Input: part model. Units: mm. Frame: model coordinates. A direction names the side the tool comes from. Give positions to 0.01 mm unless a question says otherwise; leave off trailing zeros. Write each loop counter-clockwise with the first axis right and the second up, starting at its lowest first coordinate (ties: lowest second). Pieces come first, ordered by that corner, then holes. Notation, with made-up numbers: (62.5, -22.75) -> (94.5, -22.75) arc R29 ccw to (94.5, 13.25) -> close; hole circle Ø1 at (72.25, 51.25). An arc over 180 degrees is marked (long way). Return JSON: item names as keys, results as strings. Group by question number.
Item 1: Line query: line 1 (X direction, y = 0, z = 25); line 2 (X direction, y = 29.5, z = 1); line 3 (X direction, y = 0, z = 15). Output: solid intervals per line, ascending. Write a range as [from, to].
Item 2: Set-up query: faces 4 (the face through (33.79, 0.41, -3.15)), 5 (the face through (39.962, -17, -17)), 6 (the face through (31.618, -17, 17)). Return all of +Z, -Z, +X, -X, +Y, -Y with unobstructed straight access to the full face (end or side cutting, diameter ignored); none if empty.
Item 3: Section C-C, the plane x = 47. Return loops of the section in (y, z) (3 decimals).
Item 4: Section B-B, the plane x = 28.5. Return loops of the section in (y, z) (3 decimals).
Item 5: Mould query, pull axis X, two halves, no side actions, for faces 1 (the face through (26.68, 13.65, -14.89)), 2 (the face through (38.82, -0.95, 19.44)), 3 (the face through (11.521, -10.465, -2.324)). Classes: released by +X, released by -X, zero draft, split by the parting line, or undercut.
Item 6: Section D-D, the plane y = -26. Return loops of the section in (x, z), then the cut area to 3 significant figures.
Item 7: Section A-A, the plane y = 0. Return loops of the section in (x, z) (1 decimal).
Item 8: Pin query (flat end, axial travel): P1, Ø8, axis at x = 30, z = -4, coming from the +Y side; P2, Ø1, axis at x = 38.5, y = -30.5, coming from the -Z side; P3, Ø2, axis at x = 51, z = -2, coming from the +Y side. Return the tip coordinate at first contact, or that it passes through.
from build123d import *

# Parameters (mm, degrees)
F4_D     = 6.35
F4_DEPTH = 39.4386441836
F5_D     = 6.35


with BuildPart() as f1:
    # F0 (on Front) → F1 (revolve)
    with BuildSketch(Plane.XZ):
        Polygon((10.9917372465, 10.2357640862), (10.9917372465, 0), (55.9533685446, 0), (55.9533685446, 10.2357640862), (39.9618595839, 21.1285278201), (39.9618595839, 39.4376441836), (31.6184610128, 39.4376441836), (31.6184610128, 20.2014818788), (21.8845009804, 20.2014818788), align=None)
    revolve(axis=Axis((33.4725528955, 0, 0), (-1, 0, 0)))

    # F4 (through all, one way)
    with BuildSketch(Plane(origin=(0, 0, 0), x_dir=(1, 0, 0), z_dir=(0, 0, -1))):
        with Locations((35.7924923301, 0)):
            Circle(F4_D / 2)
    extrude(amount=-F4_DEPTH, mode=Mode.SUBTRACT)

    # F5 (through all)
    with Locations(Plane(origin=(0, 0, 0), x_dir=(0, 1, 0), z_dir=(-1, 0, 0))):
        with Locations((0, 0)):
            Hole(F5_D / 2)


solid = f1.part
Answer below:
{
 "1": {"line 1": "x = [31.62, 32.62], [38.97, 39.96]", "line 2": "x = [31.62, 39.96]", "line 3": "x = [16.2, 32.62], [38.97, 48.96]"},
 "2": {"face 4": "+X, -X", "face 5": "+X", "face 6": "-X"},
 "3": {"outline": "circle Ø32.669 at (0, 0); hole circle Ø6.35 at (0, 0)"},
 "4": {"outline": "circle Ø40.403 at (0, 0); hole circle Ø6.35 at (0, 0)"},
 "5": {"face 1": "zero draft", "face 2": "undercut", "face 3": "released by -X"},
 "6": {"outline": "(31.62, -29.65) -> (39.96, -29.65) -> (39.96, 29.65) -> (31.62, 29.65) -> close", "area": "495 mm2"},
 "7": {"outline": "(11, -10.2) -> (21.9, -20.2) -> (31.6, -20.2) -> (31.6, -39.4) -> (40, -39.4) -> (40, -21.1) -> (56, -10.2) -> (56, -3.2) -> (11, -3.2) -> close; (11, 3.2) -> (32.6, 3.2) -> (32.6, 39.4) -> (31.6, 39.4) -> (31.6, 20.2) -> (21.9, 20.2) -> (11, 10.2) -> close; (39, 3.2) -> (56, 3.2) -> (56, 10.2) -> (40, 21.1) -> (40, 39.4) -> (39, 39.4) -> close"},
 "8": {"P1": "stops at y = 39.44", "P2": "stops at z = -25.6", "P3": "stops at y = 14.16"}
}
